Here's how the part is built. I have some questions about the finished solid (model axes, mm). A direction names the side the tool comes from. Round coordinates to 2 decimals unless told otherwise and drop trailing zeros. Loops run counter-clockwise (first coordinate to the right, second up) from the corner with the lowest first, then second, coordinate; pieces in that order, holes last. Notation, with made-up numbers: M -33,68 L 18,68 A21 cw 18,83 Z; hole C -38,-11.5 d5. An arc over 180 degrees is marked long. Use a Markdown table: item, result.
from build123d import *

# Parameters (mm, degrees)
SKETCH1_W               = 72.11
SKETCH1_H               = 97.4
BOSS_EXTRUDE1_DEPTH     = 2.5
SKETCH2_W               = 5
SKETCH2_H               = 97.4
BOSS_EXTRUDE2_DEPTH     = 6.375
CUT_EXTRUDE1_DEPTH      = 62.240661737
CUT_EXTRUDE1_DEPTH_BACK = 62.240661737
SKETCH3_W               = 40
SKETCH3_H               = 62


with BuildPart() as part:
    # Sketch1 → Boss-Extrude1 (new, symmetric)
    with BuildSketch(Plane(origin=(0, 0, 0), x_dir=(1, 0, 0), z_dir=(0, 1, 0))):
        Rectangle(SKETCH1_W, SKETCH1_H)
    extrude(amount=BOSS_EXTRUDE1_DEPTH, both=True)

    # Sketch2 → Boss-Extrude2 (add, symmetric)
    with BuildSketch(Plane(origin=(0, 0, 0), x_dir=(1, 0, 0), z_dir=(0, 1, 0))):
        with Locations((-33.555, 0)):
            Rectangle(SKETCH2_W, SKETCH2_H)
        with Locations((33.555, 0)):
            Rectangle(SKETCH2_W, SKETCH2_H)
    extrude(amount=BOSS_EXTRUDE2_DEPTH, both=True)

    # Sketch3 → Cut-Extrude1 (cut, two sides: drawn at the far end of the back side and taken through both)
    with BuildSketch(Plane(origin=(0, 2.5, 0), x_dir=(1, 0, 0), z_dir=(0, 1, 0)).offset(-CUT_EXTRUDE1_DEPTH_BACK)):
        Rectangle(SKETCH3_W, SKETCH3_H)
    extrude(amount=CUT_EXTRUDE1_DEPTH + CUT_EXTRUDE1_DEPTH_BACK, mode=Mode.SUBTRACT)

    # Sketch4 → Revolve1 (revolve)
    with BuildSketch(Plane(origin=(0, 0, 0), x_dir=(1, 0, 0), z_dir=(0, 1, 0)), mode=Mode.PRIVATE) as revolve1_sk:
        Polygon((20, 31), (15.058430503, 33.414723774), (30.424854519, 64.86107512), (35.366424016, 62.446351346), align=None)
    revolve1 = revolve(revolve1_sk.sketch.rotate(Axis((20, 0, -31), (0.4390406861851917, 0, -0.8984671813004836)), 180), axis=Axis((20, 0, -31), (0.4390406861851917, 0, -0.8984671813004836)))

    # Mirror1: Revolve1 across plane
    add(revolve1.mirror(Plane.XY))


solid = part.part
1. Imagine slicing it at B-B, the plane z = -0.5. Write out the boundary of the cut face in (x, y) (3 decimals), then the cut area to 3 significant figures.
Answer sheet:
| item | result |
|---|---|
| outline | M -36.055,-6.375 L -31.055,-6.375 L -31.055,-2.5 L -20,-2.5 L -20,2.5 L -31.055,2.5 L -31.055,6.375 L -36.055,6.375 Z; M 20,-2.5 L 31.055,-2.5 L 31.055,-6.375 L 36.055,-6.375 L 36.055,6.375 L 31.055,6.375 L 31.055,2.5 L 20,2.5 Z |
| area | 238 mm2 |
2. Imagine slicing it at C-C, the plane x = -23.5. Write out the boundary of the cut face in (y, z).
Answer sheet:
| item | result |
|---|---|
| outline | M -2.5,-48.7 L 2.5,-48.7 L 2.5,48.7 L -2.5,48.7 Z |
3. I need wall thicknesses on probe 1 along X at (y, z) = (3.75, -6) (3 decimals); probe 2 along X at (y, z) = (4.75, -44) (3 decimals); probe 3 along X at (y, z) = (-2.25, 2) (3 decimals). Which ranges of each line are inside material? Lowest first, please. Write a range as from..to.
Answer sheet:
| item | result |
|---|---|
| probe 1 | -36.055..-31.055, 31.055..36.055 |
| probe 2 | -36.055..-31.055, 23.267..29.438, 31.055..36.055 |
| probe 3 | -36.055..-20, 20..36.055 |
4. For pin 1 Ø5.5 at (y, z) = (0.5, -4.5) entering from +X (3 decimals); pin 2 Ø1.5 at (x, y) = (-8.5, 0) entering from -Z; pin 3 Ø3.5 at (x, z) = (25, -17) entering from -Y, each with a flat end and sliding along its axis, tell me the tip position at first contact or that it passes through.
Answer sheet:
| item | result |
|---|---|
| pin 1 | x = 36.055 |
| pin 2 | z = -48.7 |
| pin 3 | y = -2.5 |
5. Imagine slicing it at A-A, the plane x = 2.5. Write out the boundary of the cut face in (y, z).
Answer sheet:
| item | result |
|---|---|
| outline | M -2.5,-48.7 L 2.5,-48.7 L 2.5,-31 L -2.5,-31 Z; M -2.5,31 L 2.5,31 L 2.5,48.7 L -2.5,48.7 Z |
6. We'd pull the mould along X, two halves only. Please class faces 1 (the face through (34, 6.375, -1)), 2 (the face through (20, -4, 31)), 3 (the face through (31.055, -4, 1)), 4 (the face through (36.055, 0, 1)): +X half, -X half, draft (parallel to the pull), parting line (faces both ways), or undercut.
Answer sheet:
| item | result |
|---|---|
| face 1 | draft |
| face 2 | undercut |
| face 3 | undercut |
| face 4 | +X half |
7. Which directions (+Z, -Z, +X, -X, +Y, -Y) give clear straight access to the entire face, cutting with the end or side of a thin tool? Please do faces 5 (the face through (25, 2.5, -1)), 6 (the face through (-31.055, 4, 1)), 7 (the face through (20, 0, 0)).
Answer sheet:
| item | result |
|---|---|
| face 5 | +Y |
| face 6 | +Z, -Z, +Y |
| face 7 | +Y, -Y |
